```python
from build123d import *

# Parameters (mm, degrees)
SKIZZE1_W                       = 554
SKIZZE1_H                       = 1.2
SKIZZE2_W                       = 2
SKIZZE2_H                       = 0.603863108
AUFSATZ_LINEAR_AUSTRAGEN1_DEPTH = 10


with BuildPart() as part:
    # Skizze1 → Rotation1 (revolve)
    with BuildSketch(Plane.XY):
        with Locations((277, 8.925)):
            Rectangle(SKIZZE1_W, SKIZZE1_H)
    revolve(axis=Axis((0, 0, 0), (1, 0, 0)))

    # Skizze2 → Aufsatz-Linear austragen1 (add)
    with BuildSketch(Plane.ZY):
        with Locations((-7.687386884, 0)):
            Rectangle(SKIZZE2_W, SKIZZE2_H)
    extrude(amount=-AUFSATZ_LINEAR_AUSTRAGEN1_DEPTH)


solid = part.part
```
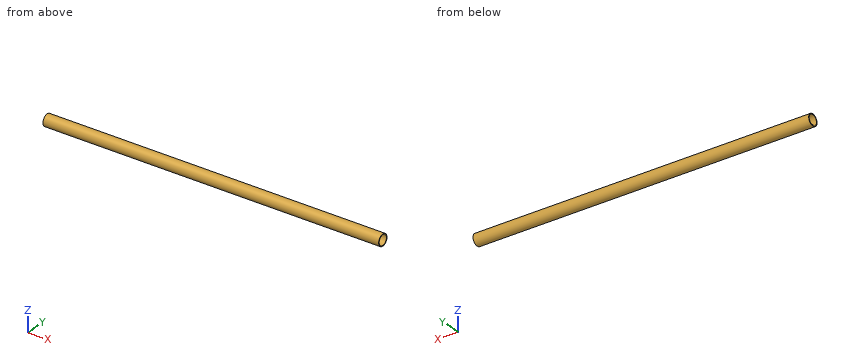
CAD build for the part. Positions are in the model's coordinates, mm. Give positions to 0.01 mm unless a question says otherwise; leave off trailing zeros. Order: outer loops, then holes, each group sorted by start corner. A loop starts at its lowest first (then second) coordinate and runs counter-clockwise, first axis right, second up. Notation, with made-up numbers: M 36.5,4 L 42.5,4 A20 cw 42.5,27 Z; hole C 25.25,-15 d11. An arc over 180 degrees is marked long. Put each result on its own line as item: value. Start each with the question number.
(1) Saw through at A-A, the plane z = 0. Write the cut outline in (x, y) (3 decimals), then the cut area to 3 significant figures.
(2) Flat gauge pins, fed straight in: pin 1 Ø10 at (y, z) = (-2, -1) entering from -X; pin 2 Ø0.5 at (y, z) = (0, -8) entering from +X; pin 3 Ø4 at (x, y) = (89.5, 4.5) entering from +Z; pin 4 Ø8 at (x, y) = (495, -4.5) entering from +Z. Where does each tip first touch, or does it go through?
(3) Saw through at B-B, the plane y = -4.5. Write the cut outline in (x, z), then the cut area to 3 significant figures.
(4) Saw through at C-C, the plane x = 354. Write the cut outline in (y, z) (3 decimals).
(5) Drill centre lines: line 1 along Y through (x, z) = (161, -0.25); line 2 along Z through (x, y) = (269.5, -1.25); line 3 along Z through (x, y) = (315, 0) (3 decimals). Where is each one in solid material? Low to high.
Check result:
1. outline: M 0,-9.525 L 554,-9.525 L 554,-8.325 L 0,-8.325 Z; M 0,8.325 L 554,8.325 L 554,9.525 L 0,9.525 Z
1. area: 1,330 mm2
2. pin 1: passes through
2. pin 2: stops at x = 10
2. pin 3: stops at z = 9.19
2. pin 4: stops at z = 9.51
3. outline: M 0,-8.39 L 554,-8.39 L 554,-7 L 0,-7 Z; M 0,7 L 554,7 L 554,8.39 L 0,8.39 Z
3. area: 1,540 mm2
4. outline: C 0,0 d19.05; hole C 0,0 d16.65
5. line 1: y = -9.52 to -8.32, 8.32 to 9.52
5. line 2: z = -9.44 to -8.23, 8.23 to 9.44
5. line 3: z = -9.525 to -8.325, 8.325 to 9.525
